```python
from build123d import *

# Parameters (mm, degrees)
SKETCH1_R                = 16.5
SKETCH1_R_2              = 12.6
BOSS_EXTRUDE1_DEPTH      = 15
BOSS_EXTRUDE2_START      = 5
SKETCH2_R                = 16.5
BOSS_EXTRUDE2_DEPTH      = 5
BOSS_EXTRUDE3_REACH      = 42.66
BOSS_EXTRUDE3_END_RADIUS = 16.5
SKETCH3_R                = 4.5
CUT_EXTRUDE1_REACH       = 42.66
CUT_EXTRUDE1_END_RADIUS  = 12.6
SKETCH4_R                = 1.6
CIRPATTERN1_COUNT        = 2
CHAMFER1_SIZE            = 0.5
SKETCH5_R                = 2.75
BOSS_EXTRUDE4_DEPTH      = 6


with BuildPart() as part:
    # Sketch1 → Boss-Extrude1 (new body)
    with BuildSketch(Plane.XY):
        Circle(SKETCH1_R)
        Circle(SKETCH1_R_2, mode=Mode.SUBTRACT)
    extrude(amount=BOSS_EXTRUDE1_DEPTH)

    # Sketch2 → Boss-Extrude2 (add)
    with BuildSketch(Plane(origin=(0, 0, 0), x_dir=(-1, 0, 0), z_dir=(0, 0, -1)).offset(BOSS_EXTRUDE2_START)):
        Circle(SKETCH2_R)
    extrude(amount=-BOSS_EXTRUDE2_DEPTH)

    # Boss-Extrude3: up to this cylinder (the profile starts outside it)
    boss_extrude3_end = Plane(origin=(0, 0, 7.5), z_dir=(0, 0, -1)) * Cylinder(BOSS_EXTRUDE3_END_RADIUS, 119.32, mode=Mode.PRIVATE)
    # Sketch3 → Boss-Extrude3 (add, up to the surface)
    with BuildSketch(Plane(origin=(0, 17.5, 0), x_dir=(1, 0, 0), z_dir=(0, 1, 0)), mode=Mode.PRIVATE) as boss_extrude3_sk1:
        with Locations(Location((0, -7.5, 0), (0, 0, 270))):
            Circle(SKETCH3_R)
    boss_extrude3_tool1 = extrude(boss_extrude3_sk1.sketch, amount=-BOSS_EXTRUDE3_REACH, mode=Mode.PRIVATE) - boss_extrude3_end
    boss_extrude3 = boss_extrude3_tool1.solids().sort_by_distance((0, 17.5, 7.5))[0]
    add(boss_extrude3)

    # Cut-Extrude1: up to this cylinder (the profile starts outside it)
    cut_extrude1_end = Plane(origin=(0, 0, 7.5), z_dir=(0, 0, -1)) * Cylinder(CUT_EXTRUDE1_END_RADIUS, 111.52, mode=Mode.PRIVATE)
    # Sketch4 → Cut-Extrude1 (cut, up to the surface)
    with BuildSketch(Plane(origin=(0, 17.5, 0), x_dir=(1, 0, 0), z_dir=(0, 1, 0)), mode=Mode.PRIVATE) as cut_extrude1_sk1:
        with Locations(Location((0, -7.5, 0), (0, 0, 270))):
            Circle(SKETCH4_R)
    cut_extrude1_tool1 = extrude(cut_extrude1_sk1.sketch, amount=-CUT_EXTRUDE1_REACH, mode=Mode.PRIVATE) - cut_extrude1_end
    cut_extrude1 = cut_extrude1_tool1.solids().sort_by_distance((0, 17.5, 7.5))[0]
    add(cut_extrude1, mode=Mode.SUBTRACT)

    # CirPattern1: Boss-Extrude3, Cut-Extrude1 ×2 about axis
    cirpattern1_axis = Axis((0, 0, 15), (0, 0, 1))
    add([boss_extrude3.rotate(cirpattern1_axis, i * 360 / CIRPATTERN1_COUNT) for i in range(1, CIRPATTERN1_COUNT)])
    add([cut_extrude1.rotate(cirpattern1_axis, i * 360 / CIRPATTERN1_COUNT) for i in range(1, CIRPATTERN1_COUNT)], mode=Mode.SUBTRACT)

    # Chamfer1
    chamfer1_edges = [part.edges().sort_by_distance(p)[0] for p in [
        (0, 17.5, 5.9),
        (0, -17.5, 5.9),
    ]]
    chamfer(chamfer1_edges, length=CHAMFER1_SIZE)

    # Sketch5 → Boss-Extrude4 (add)
    with BuildSketch(Plane(origin=(0, 0, -5), x_dir=(-1, 0, 0), z_dir=(0, 0, -1))):
        with BuildLine():
            Line((26.573684211, 6.677522556), (6.426315789, 15.197120299))
            ThreePointArc((6.426315789, 15.197120299), (0, 16.5), (-6.426315789, 15.197120299))
            Line((-6.426315789, 15.197120299), (-26.573684211, 6.677522556))
            ThreePointArc((-26.573684211, 6.677522556), (-31, 0), (-26.573684211, -6.677522556))
            Line((-26.573684211, -6.677522556), (-6.426315789, -15.197120299))
            ThreePointArc((-6.426315789, -15.197120299), (0, -16.5), (6.426315789, -15.197120299))
            Line((6.426315789, -15.197120299), (26.573684211, -6.677522556))
            ThreePointArc((26.573684211, -6.677522556), (31, 0), (26.573684211, 6.677522556))
        make_face()
        with Locations((23.75, 0)):
            Circle(SKETCH5_R, mode=Mode.SUBTRACT)
        with Locations((-23.75, 0)):
            Circle(SKETCH5_R, mode=Mode.SUBTRACT)
    extrude(amount=-BOSS_EXTRUDE4_DEPTH)


solid = part.part
```
CAD build for the part. Positions are in the model's coordinates, mm. A direction names the side the tool comes from. Coordinates: 2 decimals unless noted, no trailing zeros. Write each loop counter-clockwise with the first axis right and the second up, starting at its lowest first coordinate (ties: lowest second). Pieces come first, ordered by that corner, then holes.
(1) Flat gauge pins, fed straight in: pin 1 (7 mm diameter, centred on x = -23.75, y = 0, fed in from -Z); pin 2 (3 mm diameter, centred on y = 0.5, z = 7, fed in from +X); pin 3 (4 mm diameter, centred on x = 0, z = 7.5, fed in from +Y); pin 4 (3 mm diameter, centred on y = 1.5, z = 6.5, fed in from -X). Where does each tip first touch, or does it go through?
(2) Cut at D-D, the plane x = -22.5. List the corners of the cut face in (y, z).
(3) 3-axis set-ups, long thin cutter, end or side, ignore diameter. For faces 1 (the face through (0, -17, 3)), 2 (the face through (0, 17, 3)), 3 (the face through (0, 0, 1)): which of +Z, -Z, +X, -X, +Y, -Y reach the whole face in a straight line?
(4) Cut at A-A, the plane y = 0. List the corners of the cut face in (x, z).
(5) Cut at B-B, the plane x = 0. List the corners of the cut face in (y, z), and give its area (3 significant figures).
(6) Two-plate mould, pull along Y, no slides. Class faces 4 (the face through (-31, 0, -2)), 5 (the face through (0, 0, -5)), 6 (the face through (-9.999, -7.667, 7.902)): +Y half, -Y half, draft (parallel to the pull), parting line (faces both ways), or undercut.
(7) Drill centre lines: probe 1 along Z at (x, y) = (0, -15.35); probe 2 along Z at (x, y) = (19.5, 7); probe 3 along Y at (x, z) = (-7, 3.5). Where is each one in solid material? Low to high.
(8) Cut at C-C, the plane z = 7.5. List the corners of the cut face in (x, y).
Geometry says:
1. pin 1: stops at z = -5
1. pin 2: stops at x = 16.5
1. pin 3: stops at y = 17.4
1. pin 4: stops at x = -16.5
2. outline: (-8.4, -5) - (-2.45, -5) - (-2.45, 1) - (-8.4, 1) - close; (2.45, -5) - (8.4, -5) - (8.4, 1) - (2.45, 1) - close
3. face 1: -Y
3. face 2: +Y
3. face 3: +Z
4. outline: (-31, -5) - (-26.5, -5) - (-26.5, 1) - (-31, 1) - close; (-21, -5) - (21, -5) - (21, 1) - (16.5, 1) - (16.5, 15) - (12.6, 15) - (12.6, 1) - (-12.6, 1) - (-12.6, 15) - (-16.5, 15) - (-16.5, 1) - (-21, 1) - close; (26.5, -5) - (31, -5) - (31, 1) - (26.5, 1) - close
5. outline: (-17.5, 3) - (-16.5, 3) - (-16.5, -5) - (16.5, -5) - (16.5, 3) - (17.5, 3) - (17.5, 5.4) - (17, 5.9) - (12.6, 5.9) - (12.6, 1) - (-12.6, 1) - (-12.6, 5.9) - (-17, 5.9) - (-17.5, 5.4) - close; (-17.5, 9.6) - (-17, 9.1) - (-12.6, 9.1) - (-12.6, 15) - (-16.5, 15) - (-16.5, 12) - (-17.5, 12) - close; (12.6, 9.1) - (17, 9.1) - (17.5, 9.6) - (17.5, 12) - (16.5, 12) - (16.5, 15) - (12.6, 15) - close
5. area: 293 mm2
6. face 4: parting line
6. face 5: draft
6. face 6: undercut
7. probe 1: z = -5 to 5.9, 9.1 to 15
7. probe 2: z = -5 to 1
7. probe 3: y = -14.94 to -10.48, 10.48 to 14.94
8. outline: (-4.5, -17.5) - (-2.1, -17.5) - (-1.6, -17) - (-1.6, -12.5) arc R12.6 cw to (-1.6, 12.5) - (-1.6, 17) - (-2.1, 17.5) - (-4.5, 17.5) - (-4.5, 15.87) arc R16.5 ccw to (-4.5, -15.87) - close; (1.6, -17) - (2.1, -17.5) - (4.5, -17.5) - (4.5, -15.87) arc R16.5 ccw to (4.5, 15.87) - (4.5, 17.5) - (2.1, 17.5) - (1.6, 17) - (1.6, 12.5) arc R12.6 cw to (1.6, -12.5) - close
